Can you work these out from the model? Positions are in its coordinate system, mm. A direction names the side the tool comes from. Coordinates: 2 decimals unless noted, no trailing zeros. Order: outer loops, then holes, each group sorted by start corner. A loop starts at its lowest first (then second) coordinate and runs counter-clockwise, first axis right, second up.
```python
from build123d import *

# Parameters (mm, degrees)
F1_DEPTH = 28
F2_T     = -2.7
F4_DEPTH = 25
F6_DEPTH = 25


with BuildPart() as f1:
    # F0 (on Top) → F1 (new body)
    with BuildSketch(Plane.XY):
        Polygon((0, 35), (0, 0), (35, 0), (35, 4), (4, 35), align=None)
    extrude(amount=F1_DEPTH)

    # F2
    f2_openings = [f1.faces().sort_by_distance(p)[0] for p in [
        (19.5, 19.5, 14),
        (2, 35, 14),
        (35, 2, 14),
    ]]
    offset(amount=F2_T, openings=f2_openings)

    # F3 (on face) → F4 (cut)
    with BuildSketch(Plane(origin=(0, 0, 0), x_dir=(0, -1, 0), z_dir=(-1, 0, 0))):
        with BuildLine():
            Line((-17.460573, 10.750239), (-17.539427, 10.750239))
            ThreePointArc((-17.539427, 10.750239), (-17.5, 10.75), (-17.460573, 10.750239))
        make_face()
        with BuildLine():
            Line((-21.960573, 10.750239), (-17.539427, 10.750239))
            Line((-17.539427, 10.750239), (-17.460573, 10.750239))
            Line((-17.460573, 10.750239), (-13.039427, 10.750239))
            Line((-13.039427, 10.750239), (-12.960573, 10.750239))
            ThreePointArc((-12.960573, 10.750239), (-10.688005, 11.715885), (-9.75, 14))
            Line((-9.75, 14), (-13, 14))
            Line((-13, 14), (-17.5, 14))
            Line((-17.5, 14), (-22, 14))
            Line((-22, 14), (-25.25, 14))
            ThreePointArc((-25.25, 14), (-24.311995, 11.715885), (-22.039427, 10.750239))
            Line((-22.039427, 10.750239), (-21.960573, 10.750239))
        make_face()
        with BuildLine():
            ThreePointArc((-22.039427, 10.750239), (-22, 10.75), (-21.960573, 10.750239))
            Line((-21.960573, 10.750239), (-22.039427, 10.750239))
        make_face()
        with BuildLine():
            Line((-12.960573, 10.750239), (-13.039427, 10.750239))
            ThreePointArc((-13.039427, 10.750239), (-13, 10.75), (-12.960573, 10.750239))
        make_face()
        with BuildLine():
            ThreePointArc((-21.999708, 17.25), (-24.297994, 16.2982), (-25.25, 14))
            Line((-25.25, 14), (-22, 14))
            Line((-22, 14), (-17.5, 14))
            Line((-17.5, 14), (-13, 14))
            Line((-13, 14), (-9.75, 14))
            ThreePointArc((-9.75, 14), (-10.727581, 16.323491), (-13.072222, 17.249197))
            Line((-13.072222, 17.249197), (-21.999708, 17.25))
        make_face()
    extrude(amount=-F4_DEPTH, mode=Mode.SUBTRACT)

    # F5 (on face) → F6 (cut)
    with BuildSketch(Plane.XZ):
        with BuildLine():
            Line((17.880831, 10.77239), (21.787071, 10.756983))
            ThreePointArc((21.787071, 10.756983), (25.248254, 13.893489), (21.999979, 17.25))
            Line((21.999979, 17.25), (17.513798, 17.249971))
            ThreePointArc((17.513798, 17.249971), (17.499979, 17.25), (17.48616, 17.249971))
            Line((17.48616, 17.249971), (13.019522, 17.249941))
            ThreePointArc((13.019522, 17.249941), (12.999979, 17.25), (12.980436, 17.249941))
            ThreePointArc((12.980436, 17.249941), (9.760165, 14.256843), (12.46861, 10.793737))
            Line((12.46861, 10.793737), (13.506082, 10.789645))
            Line((13.506082, 10.789645), (17.093721, 10.775494))
            Line((17.093721, 10.775494), (17.880831, 10.77239))
        make_face()
        with BuildLine():
            ThreePointArc((17.093721, 10.775494), (17.487181, 10.750025), (17.880831, 10.77239))
            Line((17.880831, 10.77239), (17.093721, 10.775494))
        make_face()
        with BuildLine():
            ThreePointArc((12.46861, 10.793737), (12.987181, 10.750025), (13.506082, 10.789645))
            Line((13.506082, 10.789645), (12.46861, 10.793737))
        make_face()
    extrude(amount=-F6_DEPTH, mode=Mode.SUBTRACT)


solid = f1.part
```
1. On a 3-axis mill with a long thin cutter (end or side, diameter ignored), from which of +Z, -Z, +X, -X, +Y, -Y can I reach the whole of each face in a straight line? I mean faces 1 (the flat face through (1, 15, 10.75)), 2 (the flat face through (17, 0, 8)), 3 (the flat face through (19, 2.7, 9)), 4 (the cylindrical face through (9.766, 1.331, 14.324)). Say none if no direction works.
Completed:
face 1: +X, -X
face 2: +Z, -Z, +X, -X, -Y
face 3: +X, +Y
face 4: +Y, -Y
2. Imagine slicing it at B-B on y = 26. Please give me the cut outline in (x, z), then the cut area to 3 significant figures.
Completed:
outline: (0, 0) - (13, 0) - (13, 2.7) - (2.7, 2.7) - (2.7, 25.3) - (13, 25.3) - (13, 28) - (0, 28) - close
area: 131 mm2
3. Thinking about a two-plate mould opening in Z: for faces 5 (the flat face through (15, 15, 2.7)), 6 (the flat face through (35, 2, 14)), 7 (the flat face through (13, 14, 0)), which applies, pulls with the +Z half, pulls with the -Z half, needs draft (parallel to the pull), parting line crosses it, or undercut?
Completed:
face 5: undercut
face 6: needs draft
face 7: pulls with the -Z half
4. Imagine slicing it at D-D on z = 18.75. Please give me the cut outline in (x, y).
Completed:
outline: (0, 0) - (35, 0) - (35, 2.7) - (2.7, 2.7) - (2.7, 35) - (0, 35) - close
5. I'm going to push flat-ended pins straight in: pin 1 (6 mm diameter, centred on x = 6, y = 15, fed in from -Z); pin 2 (1 mm diameter, centred on x = 27.5, z = 17, fed in from +Y); pin 3 (3 mm diameter, centred on y = 11.5, z = 15, fed in from +X). Where does each tip first touch, or does it pass through?
Completed:
pin 1: stops at z = 0
pin 2: stops at y = 2.7
pin 3: stops at x = 2.7
6. Imagine slicing it at A-A on x = 28. Please give me the cut outline in (y, z), then the cut area to 3 significant figures.
Completed:
outline: (0, 0) - (11, 0) - (11, 2.7) - (2.7, 2.7) - (2.7, 25.3) - (11, 25.3) - (11, 28) - (0, 28) - close
area: 120 mm2
7. Imagine slicing it at C-C on y = 20. Please give me the cut outline in (x, z).
Completed:
outline: (0, 0) - (19, 0) - (19, 2.7) - (2.7, 2.7) - (2.7, 10.75) - (0, 10.75) - close; (0, 17.25) - (2.7, 17.25) - (2.7, 25.3) - (19, 25.3) - (19, 28) - (0, 28) - close
8. Please list where these lines run through material, in increasing order: probe 1 along Z at (x, y) = (4.5, 15.5); probe 2 along X at (y, z) = (32, 16).
Completed:
probe 1: z = 0 to 2.7, 25.3 to 28
probe 2: x = 0 to 2.7
